Source: CAD feature listing. Evaluate the final solid. Frame: model axes, mm. Face numbers are marked on the shaded views. A direction names the side the tool comes from. Give positions to 0.01 mm unless a question says otherwise; leave off trailing zeros. Write each loop counter-clockwise with the first axis right and the second up, starting at its lowest first coordinate (ties: lowest second). Pieces come first, ordered by that corner, then holes.
Autodesk Inventor part; units mm, degrees
ref_plane "YZ Plane" through (0, 0, 0) normal (1, 0, 0) x (0, 1, 0)
ref_plane "XZ Plane" through (0, 0, 0) normal (0, 1, 0) x (-1, 0, 0)
ref_plane "XY Plane" through (0, 0, 0) normal (0, 0, 1) x (1, 0, 0)
sketch "Sketch1" plane through (0, 0, 0) normal (0, 1, 0) x (-1, 0, 0)
  line L0 (0, 0) -> (50.8, 0)
  line L1 (50.8, 0) -> (50.8, 76.2)
  line L2 (50.8, 76.2) -> (0, 76.2)
  line L3 (0, 76.2) -> (0, 0)
  circle A0 centre (35.4838, 71.755) radius 2.3813
  circle A1 centre (35.4838, 55.245) radius 2.3813
  circle A2 centre (15.1638, 71.755) radius 2.3813
  circle A3 centre (15.1638, 55.245) radius 2.3813
  line L4 (50.8, 38.1) -> (0, 38.1)
  circle A4 centre (35.4838, 4.445) radius 2.3813
  circle A5 centre (35.4838, 20.955) radius 2.3813
  circle A6 centre (15.1638, 4.445) radius 2.3813
  circle A7 centre (15.1638, 20.955) radius 2.3813
  line L5 (0, 0) -> (50.8, 0)
  line L6 (50.8, 0) -> (50.8, -6.35)
  line L7 (50.8, -6.35) -> (0, -6.35)
  line L8 (0, -6.35) -> (0, 0)
  line L9 (0, -6.35) -> (50.8, -6.35)
  line L10 (50.8, -6.35) -> (50.8, -9.525)
  line L11 (50.8, -9.525) -> (0, -9.525)
  line L12 (0, -9.525) -> (0, -6.35)
  dimension "d0" = 50.8
  dimension "d1" = 76.2
  dimension "d2" = 4.7625
  dimension "d3" = 15.3162
  dimension "d4" = 4.445
  dimension "d7" = 16.51
  dimension "d10" = 20.32
  dimension "d15" = 50.8
  dimension "d16" = 6.35
  dimension "d17" = 50.8
  dimension "d18" = 3.175
extrude "Extrusion1" add sketch "Sketch1" along normal blind 3.175
extrude "Extrusion2" add sketch "Sketch1" along normal blind 127 contours L7 L10 L11 L12
properties part number "Gripper Slider Connecting Plate & Bar"
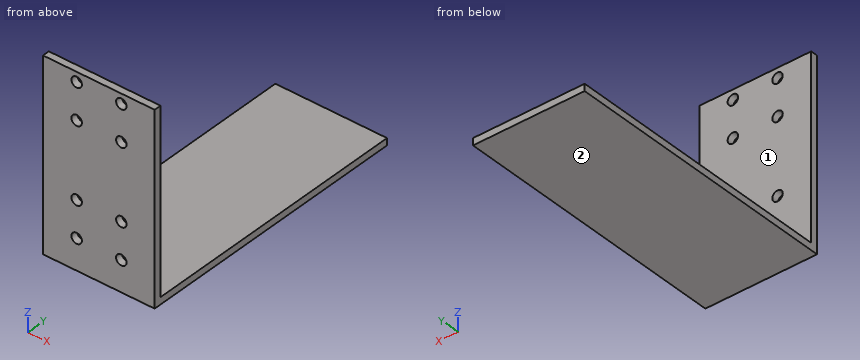
1. Line query: L1, parallel to Y at x = -28.5, z = 20.5 (3 decimals); L2, parallel to Z at x = -3, y = 49.5 (3 decimals). Output: solid intervals per line, ascending.
2. Cut plane B-B, the plane y = 31. Return the cut outline in (x, z) (3 decimals).
3. Cut plane A-A, the plane x = -22. Return the cut outline in (y, z) (3 decimals), then the cut area to 3 significant figures.
4. Cut plane C-C, the plane z = 43.5. Return the cut outline in (x, y) (3 decimals).
5. Access query for the marked faces 1 and 2. Directions: +Z, -Z, +X, -X, +Y, -Y. A direction counts if a zero-diameter tool reaches every point of the face in a straight line with its end or side. Return the directions, or none.
6. Contact query for flat-ended pins moving along their axis: P1, Ø5.5, axis at x = -15.16, z = 55.24, coming from the +Y side (3 decimals); P2, Ø8, axis at x = -6.5, y = 66, coming from the +Z side. Output: stop coordinate, or through.
Response values:
1. L1: y = 0 to 3.175
1. L2: z = -9.525 to -6.35
2. outline: (-50.8, -9.525) - (0, -9.525) - (0, -6.35) - (-50.8, -6.35) - close
3. outline: (0, -9.525) - (127, -9.525) - (127, -6.35) - (3.175, -6.35) - (3.175, 76.2) - (0, 76.2) - close
3. area: 665 mm2
4. outline: (-50.8, 0) - (0, 0) - (0, 3.175) - (-50.8, 3.175) - close
5. face 1: +Z, +X, -X, +Y
5. face 2: -Z, +X, -X, +Y, -Y
6. P1: stops at y = 3.175
6. P2: stops at z = -6.35
